Geometry check sheet. Reference: the model listing, model coordinates, mm. Face numbers are marked on the shaded views. Round coordinates to 2 decimals unless told otherwise and drop trailing zeros. Write each loop counter-clockwise with the first axis right and the second up, starting at its lowest first coordinate (ties: lowest second). Pieces come first, ordered by that corner, then holes. Notation, with made-up numbers: (31.5, 26) -> (64.5, 26) arc R18 cw to (64.5, 51) -> close; hole circle Ø7 at (80, -40). An arc over 180 degrees is marked (long way). Use a Markdown table: item, result.
```python
from build123d import *

# Parameters (mm, degrees)
SKETCH1_R           = 3
SKETCH1_R_2         = 2
BOSS_EXTRUDE1_DEPTH = 38
SKETCH2_R           = 5
SKETCH2_R_2         = 3
BOSS_EXTRUDE2_DEPTH = 2
BOSS_EXTRUDE3_START = -2
SKETCH3_R           = 5
SKETCH3_R_2         = 3
BOSS_EXTRUDE3_DEPTH = 2
FILLET4_R           = 1
FILLET5_R           = 1
FILLET6_R           = 1


with BuildPart() as part:
    # Sketch1 → Boss-Extrude1 (new body)
    with BuildSketch(Plane(origin=(0, 0, 0), x_dir=(1, 0, 0), z_dir=(0, 1, 0))):
        with Locations(Location((0, 0, 0), (0, 0, 270))):
            Circle(SKETCH1_R)
        with Locations(Location((0, 0, 0), (0, 0, 270))):
            Circle(SKETCH1_R_2, mode=Mode.SUBTRACT)
    extrude(amount=BOSS_EXTRUDE1_DEPTH)

    # Sketch2 → Boss-Extrude2 (add)
    with BuildSketch(Plane.XZ):
        with Locations(Location((0, 0, 0), (0, 0, 270))):
            Circle(SKETCH2_R)
        with Locations(Location((0, 0, 0), (0, 0, 270))):
            Circle(SKETCH2_R_2, mode=Mode.SUBTRACT)
    extrude(amount=-BOSS_EXTRUDE2_DEPTH)

    # Sketch3 → Boss-Extrude3 (add)
    with BuildSketch(Plane(origin=(0, 38, 0), x_dir=(1, 0, 0), z_dir=(0, 1, 0)).offset(BOSS_EXTRUDE3_START)):
        with Locations(Location((0, 0, 0), (0, 0, 90))):
            Circle(SKETCH3_R)
        with Locations(Location((0, 0, 0), (0, 0, 90))):
            Circle(SKETCH3_R_2, mode=Mode.SUBTRACT)
    extrude(amount=BOSS_EXTRUDE3_DEPTH)

    # Fillet4
    fillet4_edges = [part.edges().sort_by_distance(p)[0] for p in [
        (0, 0, 5),
    ]]
    fillet(fillet4_edges, radius=FILLET4_R)

    # Fillet5
    fillet5_edges = [part.edges().sort_by_distance(p)[0] for p in [
        (0, 2, 5),
    ]]
    fillet(fillet5_edges, radius=FILLET5_R - 0.0001)  # a hair under: the kernel refuses the full size

    # Fillet6
    fillet6_edges = [part.edges().sort_by_distance(p)[0] for p in [
        (0, 36, 5),
        (0, 38, 5),
    ]]
    fillet(fillet6_edges, radius=FILLET6_R - 0.0001)  # a hair under: the kernel refuses the full size


solid = part.part
```
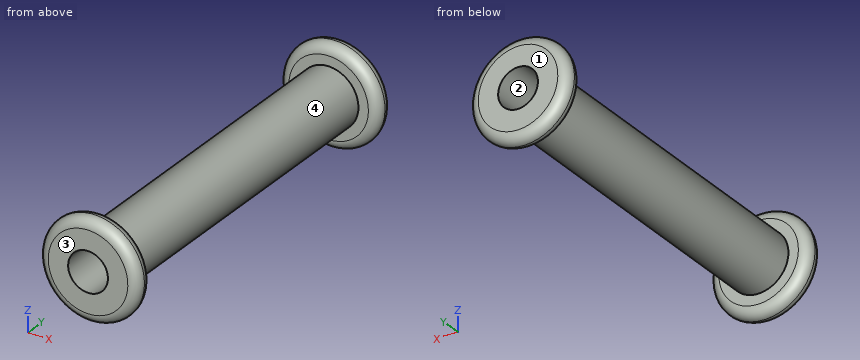
(1) Thickness scan on line 1 (X direction, y = 16, z = 0); line 2 (Y direction, x = -3.5, z = -1.25); line 3 (X direction, y = 18.5, z = -0.75). Record the ranges inside material, lowest first.
A:
| item | result |
|---|---|
| line 1 | x = -3 to -2, 2 to 3 |
| line 2 | y = 0 to 2, 36 to 38 |
| line 3 | x = -2.9 to -1.85, 1.85 to 2.9 |
(2) Gauge pin test, flat ends, axial feed: pin 1 Ø4 at (x, y) = (3.5, 6.5) entering from +Z; pin 2 Ø1 at (y, z) = (21.5, 2) entering from +X; pin 3 Ø1.5 at (x, y) = (2.5, 33.5) entering from -Z; pin 4 Ø3.5 at (x, z) = (0, 0) entering from -Y. Record the tip position at first contact, or that the pin passes through.
A:
| item | result |
|---|---|
| pin 1 | stops at z = 2.6 |
| pin 2 | stops at x = 2.6 |
| pin 3 | stops at z = -2.44 |
| pin 4 | passes through |
(3) Section check C-C on y = 5. Record the cut outline in (x, z), plus the area to 3 significant figures.
A:
| item | result |
|---|---|
| outline | circle Ø6 at (0, 0); hole circle Ø4 at (0, 0) |
| area | 15.7 mm2 |
(4) Release check for a two-part mould opening along Y. For the marked faces 1, 2, 3 and 4 record: +Y half, -Y half, draft (parallel to the pull), parting line (faces both ways), or undercut.
A:
| item | result |
|---|---|
| face 1 | +Y half |
| face 2 | draft |
| face 3 | -Y half |
| face 4 | undercut |
